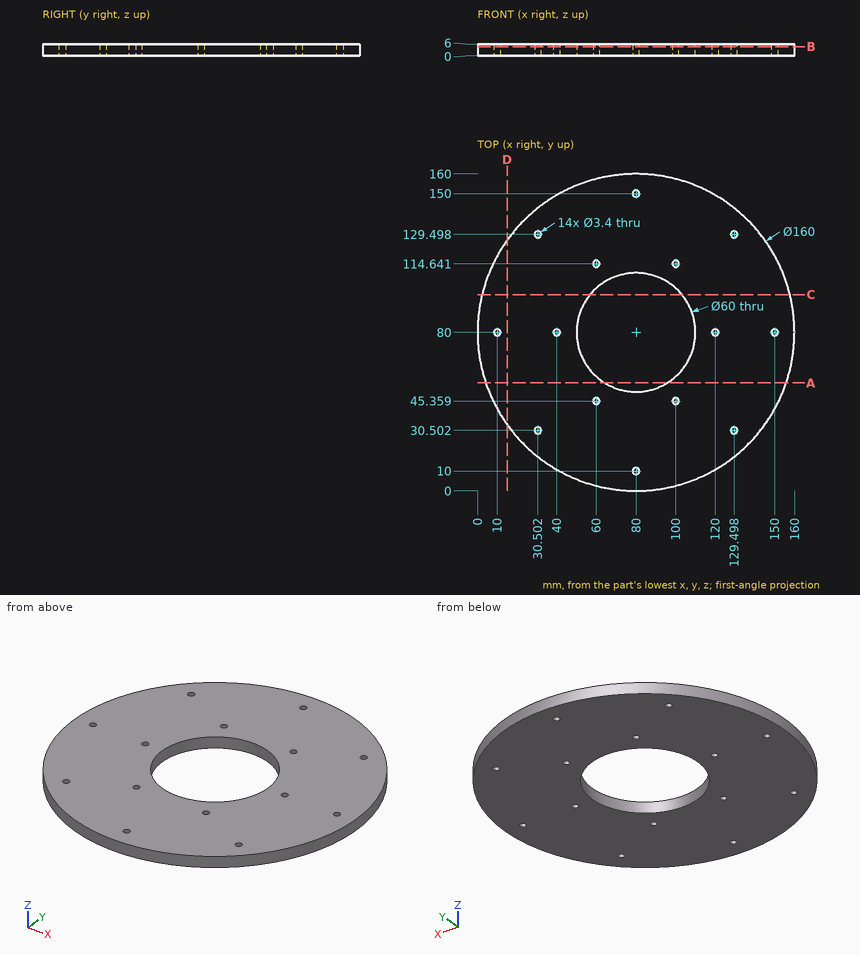
Geometry: see drawing. Coordinates: mm, zero at the bounding-box minimum. Round coordinates to 2 decimals unless told otherwise and drop trailing zeros. Write each loop counter-clockwise with the first axis right and the second up, starting at its lowest first coordinate (ties: lowest second). Pieces come first, ordered by that corner, then holes.
1) Ray query, L1, parallel to Y at x = 131, z = 1.05 (1 decimal); L2, parallel to Y at x = 100, z = 1.5; L3, parallel to X at y = 100.5, z = 1.55 (1 decimal). Return the intervals inside material, ascending.
2) Cut plane D-D (x = 15). Return the cut outline in (y, z).
3) Cut plane A-A (y = 54.5). Return the cut outline in (x, z).
4) Contact query for flat-ended pins moving along their axis: P1, Ø2, axis at x = 129.5, y = 129.5, coming from the +Z side; P2, Ø8, axis at x = 130, y = 142.5, coming from the -Z side; P3, Ø1.5, axis at x = 77.5, z = 1, coming from the -Y side; P4, Ø1, axis at y = 40.5, z = 3.5, coming from the -X side. Output: stop coordinate, or through.
5) Cut plane C-C (y = 99). Return the cut outline in (x, z).
6) Cut plane B-B (z = 4.65). Count the separate pieces of the cut face and the enclosed holes in it, then the cut area to 3 significant figures.
Geometry says:
1. L1: y = 18.4 to 29.7, 31.3 to 128.7, 130.3 to 141.6
1. L2: y = 2.54 to 43.66, 47.06 to 57.64, 102.36 to 112.94, 116.34 to 157.46
1. L3: x = 2.7 to 58.1, 101.9 to 157.3
2. outline: (33.36, 0) - (126.64, 0) - (126.64, 6) - (33.36, 6) - close
3. outline: (4.17, 0) - (64.2, 0) - (64.2, 6) - (4.17, 6) - close; (95.8, 0) - (155.83, 0) - (155.83, 6) - (95.8, 6) - close
4. P1: passes through
4. P2: stops at z = 0
4. P3: stops at y = 0.02
4. P4: stops at x = 10.15
5. outline: (2.29, 0) - (56.78, 0) - (56.78, 6) - (2.29, 6) - close; (103.22, 0) - (157.71, 0) - (157.71, 6) - (103.22, 6) - close
6. separate pieces: 1
6. enclosed holes: 15
6. area: 17,200 mm2
